Design review of the part built by this model. Coordinates are the model's own, in mm. Coordinates: 2 decimals unless noted, no trailing zeros. Loops run counter-clockwise (first coordinate to the right, second up) from the corner with the lowest first, then second, coordinate; pieces in that order, holes last.
from build123d import *

# Parameters (mm, degrees)
SKETCH2_W           = 101.6
SKETCH2_H           = 280
BOSS_EXTRUDE1_DEPTH = 25.4
SKETCH3_R           = 6
CUT_EXTRUDE1_DEPTH  = 25.4
SKETCH4_R           = 16
CUT_EXTRUDE2_DEPTH  = 25.4


with BuildPart() as part:
    # Sketch2 → Boss-Extrude1 (new body)
    with BuildSketch(Plane(origin=(0, 0, 0), x_dir=(1, 0, 0), z_dir=(0, 1, 0))):
        with Locations((50.8, 140)):
            Rectangle(SKETCH2_W, SKETCH2_H)
    extrude(amount=BOSS_EXTRUDE1_DEPTH)

    # Sketch3 → Cut-Extrude1 (cut)
    with BuildSketch(Plane(origin=(0, 25.4, 0), x_dir=(1, 0, 0), z_dir=(0, 1, 0))):
        with Locations((71, 265)):
            Circle(SKETCH3_R)
        with Locations((31, 265)):
            Circle(SKETCH3_R)
        with Locations((31, 185)):
            Circle(SKETCH3_R)
        with Locations((71, 185)):
            Circle(SKETCH3_R)
    extrude(amount=-CUT_EXTRUDE1_DEPTH, mode=Mode.SUBTRACT)

    # Sketch4 → Cut-Extrude2 (cut)
    with BuildSketch(Plane(origin=(0, 25.4, 0), x_dir=(1, 0, 0), z_dir=(0, 1, 0))):
        with Locations((40, 40)):
            Circle(SKETCH4_R)
    extrude(amount=-CUT_EXTRUDE2_DEPTH, mode=Mode.SUBTRACT)


solid = part.part
Q1. Take a section at C-C, the plane y = 12.25. Write out the cut boundary in (x, z).
Q2. Take a section at A-A, the plane x = 40. Write out the cut boundary in (y, z).
Q3. Take a section at B-B, the plane z = -265. Write out the cut boundary in (x, y).
Q4. For line 1 (X direction, y = 7.5, z = -185); line 2 (X direction, y = 21.25, z = -39.5); line 3 (Z direction, x = 31, y = 8.5), list the stretches that pass through material, from the lowest coordinate up.
Q5. Take a section at D-D, the plane z = -40. Write out the cut boundary in (x, y).
Entries:
1. outline: (0, -280) - (101.6, -280) - (101.6, 0) - (0, 0) - close; hole circle Ø32 at (40, -40); hole circle Ø12 at (31, -265); hole circle Ø12 at (31, -185); hole circle Ø12 at (71, -265); hole circle Ø12 at (71, -185)
2. outline: (0, -280) - (25.4, -280) - (25.4, -56) - (0, -56) - close; (0, -24) - (25.4, -24) - (25.4, 0) - (0, 0) - close
3. outline: (0, 0) - (25, 0) - (25, 25.4) - (0, 25.4) - close; (37, 0) - (65, 0) - (65, 25.4) - (37, 25.4) - close; (77, 0) - (101.6, 0) - (101.6, 25.4) - (77, 25.4) - close
4. line 1: x = 0 to 25, 37 to 65, 77 to 101.6
4. line 2: x = 0 to 24.01, 55.99 to 101.6
4. line 3: z = -280 to -271, -259 to -191, -179 to -53.23, -26.77 to 0
5. outline: (0, 0) - (24, 0) - (24, 25.4) - (0, 25.4) - close; (56, 0) - (101.6, 0) - (101.6, 25.4) - (56, 25.4) - close
